from build123d import *

# Parameters (mm, degrees)
F0_R      = 2.5
F0_W      = 40
F0_H      = 21
F0_R_2    = 6.75
F1_DEPTH  = 6
F1_FACE_W = 60
F1_FACE_H = 6
F2_DEPTH  = 1


with BuildPart() as f1:
    # F0 (on Top) → F1 (new body)
    with BuildSketch(Plane.XY):
        Polygon((30, 16.5), (20, 16.5), (10, 16.5), (6, 20.5), (-6, 20.5), (-10, 16.5), (-20, 16.5), (-30, 16.5), (-30, 10.5), (-30, -10.5), (-30, -22.5), (-20, -22.5), (20, -22.5), (30, -22.5), (30, -10.5), (30, 10.5), align=None)
        with Locations((-9, -15.5)):
            Circle(F0_R, mode=Mode.SUBTRACT)
        with Locations((9, -15.5)):
            Circle(F0_R, mode=Mode.SUBTRACT)
        with Locations((-22.73, 0)):
            Circle(F0_R, mode=Mode.SUBTRACT)
        Rectangle(F0_W, F0_H, mode=Mode.SUBTRACT)
        with Locations((0, 15.5)):
            Circle(F0_R, mode=Mode.SUBTRACT)
        Rectangle(F0_W, F0_H)
        with Locations((-10, 0)):
            Circle(F0_R_2, mode=Mode.SUBTRACT)
        with Locations((2.73, 0)):
            Circle(F0_R, mode=Mode.SUBTRACT)
    extrude(amount=F1_DEPTH)

    # F1_face (on face) → F2 (cut)
    with BuildSketch(Plane(origin=(0, -22.5, 3), x_dir=(1, 0, 0), z_dir=(0, -1, 0))):
        Rectangle(F1_FACE_W, F1_FACE_H)
    extrude(amount=-F2_DEPTH, mode=Mode.SUBTRACT)


solid = f1.part
Source: CAD feature listing. Evaluate the final solid. Frame: model axes, mm. A direction names the side the tool comes from. Give positions to 0.01 mm unless a question says otherwise; leave off trailing zeros. Order: outer loops, then holes, each group sorted by start corner. A loop starts at its lowest first (then second) coordinate and runs counter-clockwise, first axis right, second up. Notation, with made-up numbers: (-11.75, -5.5) -> (31.25, -5.5) arc R29 cw to (31.25, 23.5) -> close; hole circle Ø6 at (1, -10). An arc over 180 degrees is marked (long way). Write item = value, one per line.
Q1. Cut plane B-B, the plane y = 15.5. Output: boundary loops of the cut face in (x, z).
Data:
outline = (-30, 0) -> (-2.5, 0) -> (-2.5, 6) -> (-30, 6) -> close; (2.5, 0) -> (30, 0) -> (30, 6) -> (2.5, 6) -> close
Q2. Set-up query: faces 4 (the face through (20, 16.5, 3)), 5 (the face through (30, -3, 3)), 6 (the face through (-20, 16.5, 3)). Return all of +Z, -Z, +X, -X, +Y, -Y with unobstructed straight access to the full face (end or side cutting, diameter ignored); none if empty.
Data:
face_4 = +Z, -Z, +X, +Y
face_5 = +Z, -Z, +X, +Y, -Y
face_6 = +Z, -Z, -X, +Y
Q3. Pull-direction query (Y, two-part tool) for faces 1 (the face through (8.46, -17.94, 2.96)), 2 (the face through (0, -21.5, 3)), 3 (the face through (0, 0, 6)); classes: released by +Y, released by -Y, zero draft, split by the parting line, or undercut.
Data:
face_1 = undercut
face_2 = released by -Y
face_3 = zero draft
Q4. Pin query (flat end, axial travel): pin 1 (3 mm diameter, centred on x = 2.73, y = 0, fed in from -Z); pin 2 (3 mm diameter, centred on x = -21, z = 2.5, fed in from +Y). Return the tip coordinate at first contact, or that it passes through.
Data:
pin_1 = through
pin_2 = 16.5
Q5. Cut plane D-D, the plane z = 4.25. Output: boundary loops of the cut face in (x, y), and give its area (3 significant figures).
Data:
outline = (-30, -21.5) -> (30, -21.5) -> (30, 16.5) -> (10, 16.5) -> (6, 20.5) -> (-6, 20.5) -> (-10, 16.5) -> (-30, 16.5) -> close; hole circle Ø5 at (-22.73, 0); hole circle Ø13.5 at (-10, 0); hole circle Ø5 at (-9, -15.5); hole circle Ø5 at (0, 15.5); hole circle Ø5 at (2.73, 0); hole circle Ø5 at (9, -15.5)
area = 2,100 mm^2
Q6. Cut plane C-C, the plane y = 0. Output: boundary loops of the cut face in (x, z).
Data:
outline = (-30, 0) -> (-25.23, 0) -> (-25.23, 6) -> (-30, 6) -> close; (-20.23, 0) -> (-16.75, 0) -> (-16.75, 6) -> (-20.23, 6) -> close; (-3.25, 0) -> (0.23, 0) -> (0.23, 6) -> (-3.25, 6) -> close; (5.23, 0) -> (30, 0) -> (30, 6) -> (5.23, 6) -> close
Q7. Material intervals for line 1 (Y direction, x = 0, z = 1.25); line 2 (X direction, y = -0.5, z = 1); line 3 (Y direction, x = -9, z = 4.05), sorted ascending. Write a range as from..to.
Data:
line_1 = -21.5..13, 18..20.5
line_2 = -30..-25.18, -20.28..-16.73, -3.27..0.28, 5.18..30
line_3 = -21.5..-18, -13..-6.68, 6.68..17.5
Q8. Cut plane A-A, the plane x = 9. Output: boundary loops of the cut face in (y, z), and give its area (3 significant figures).
Data:
outline = (-21.5, 0) -> (-18, 0) -> (-18, 6) -> (-21.5, 6) -> close; (-13, 0) -> (17.5, 0) -> (17.5, 6) -> (-13, 6) -> close
area = 204 mm^2
